The figure shows three views and two pictorial views of one solid part (mm, origin at its lowest corner). Answer the questions. A direction names the side the tool comes from. Coordinates: 2 decimals unless noted, no trailing zeros. Order: outer loops, then holes, each group sorted by start corner. A loop starts at its lowest first (then second) coordinate and runs counter-clockwise, first axis right, second up. Notation, with made-up numbers: (-5, 15) -> (19, 15) arc R15 ccw to (19, 35) -> close; hole circle Ø9 at (17, 32). An arc over 180 degrees is marked (long way). Return JSON: item names as keys, results as strings.
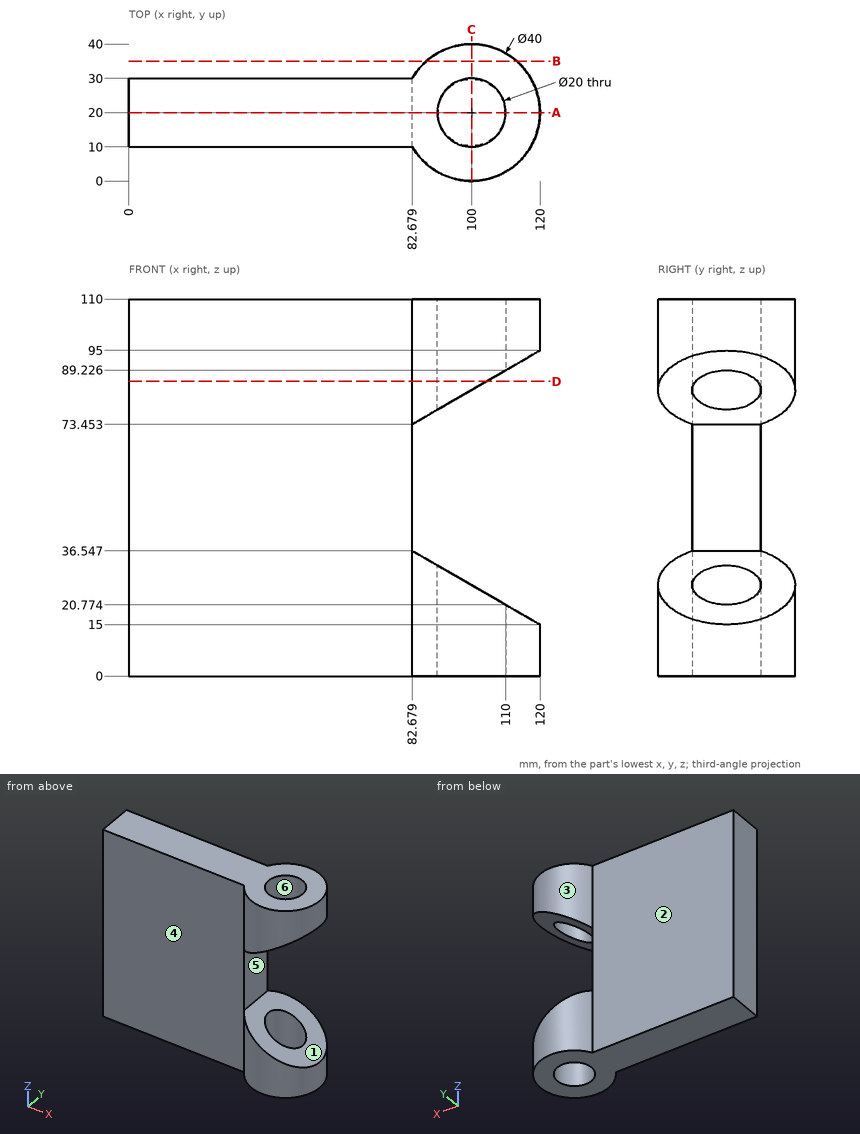
Item 1: Which of the six approach directions +Z, -Z, +X, -X, +Y, -Y give full straight-line access (tool end or side, diameter ignored) to the marked faces 1, 2 and 3?
Answer list:
{"face 1": "+X, +Y, -Y", "face 2": "+Z, -Z, -X, +Y", "face 3": "+Z, -Z"}
Item 2: Flat-ended cylindrical pins translate along their axes: pin 1 (1.5 mm diameter, centred on x = 90, z = 78, fed in from -Y); pin 2 (1 mm diameter, centred on y = 25, z = 80.5, fed in from +X); pin 3 (1.5 mm diameter, centred on y = 25.5, z = 38, fed in from +X). Find the tip coordinate at first contact, or state that the pin passes through.
Answer list:
{"pin 1": "y = 2.27", "pin 2": "x = 91.65", "pin 3": "x = 82.68"}
Item 3: The part is cut by section D-D on z = 86. Determine the outline of the cut face in (x, y) (1 decimal), plus the area to 3 significant figures.
Answer list:
{"outline": "(0, 10) -> (82.7, 10) arc R20 ccw to (104.4, 0.5) -> (104.4, 11) arc R10 cw (long way) to (104.4, 29) -> (104.4, 39.5) arc R20 ccw to (82.7, 30) -> (0, 30) -> close", "area": "2,180 mm2"}
Item 4: The part is cut by section B-B on y = 35. Determine the outline of the cut face in (x, z) (1 decimal), plus the area to 3 significant figures.
Answer list:
{"outline": "(86.8, 0) -> (113.2, 0) -> (113.2, 18.9) -> (86.8, 34.2) -> close; (86.8, 75.8) -> (113.2, 91.1) -> (113.2, 110) -> (86.8, 110) -> close", "area": "1,400 mm2"}
Item 5: Find the intervals of material crossed by probe 1 along Y at (x, z) = (100, 18); probe 2 along X at (y, z) = (20, 100.5); probe 3 along Y at (x, z) = (28, 66.5), in increasing order.
Answer list:
{"probe 1": "0 to 10, 30 to 40", "probe 2": "0 to 90, 110 to 120", "probe 3": "10 to 30"}
Item 6: The part is cut by section C-C on x = 100. Determine the outline of the cut face in (y, z), plus the area to 3 significant figures.
Answer list:
{"outline": "(0, 0) -> (10, 0) -> (10, 26.55) -> (0, 26.55) -> close; (0, 83.45) -> (10, 83.45) -> (10, 110) -> (0, 110) -> close; (30, 0) -> (40, 0) -> (40, 26.55) -> (30, 26.55) -> close; (30, 83.45) -> (40, 83.45) -> (40, 110) -> (30, 110) -> close", "area": "1,060 mm2"}
Item 7: The part is cut by section A-A on y = 20. Determine the outline of the cut face in (x, z), plus the area to 3 significant figures.
Answer list:
{"outline": "(0, 0) -> (90, 0) -> (90, 32.32) -> (82.68, 36.55) -> (82.68, 73.45) -> (90, 77.68) -> (90, 110) -> (0, 110) -> close; (110, 0) -> (120, 0) -> (120, 15) -> (110, 20.77) -> close; (110, 89.23) -> (120, 95) -> (120, 110) -> (110, 110) -> close", "area": "9,960 mm2"}
Item 8: Determine the mould class of the marked faces 4, 5 and 6 for opening direction X: pulls with the +X half, pulls with the -X half, needs draft (parallel to the pull), parting line crosses it, or undercut.
Answer list:
{"face 4": "needs draft", "face 5": "pulls with the +X half", "face 6": "undercut"}
